Could you check a few things on this drawing? It's one solid part, dimensions in mm from its lowest x, y, z. Round coordinates to 2 decimals unless told otherwise and drop trailing zeros. Write each loop counter-clockwise with the first axis right and the second up, starting at its lowest first coordinate (ties: lowest second). Pieces come first, ordered by that corner, then holes. Notation, with made-up numbers: (5.5, -10.75) -> (56.5, -10.75) arc R29 cw to (56.5, 11.25) -> close; hole circle Ø5 at (70.5, 44). An arc over 180 degrees is marked (long way). Answer in a Markdown table with one row per item.
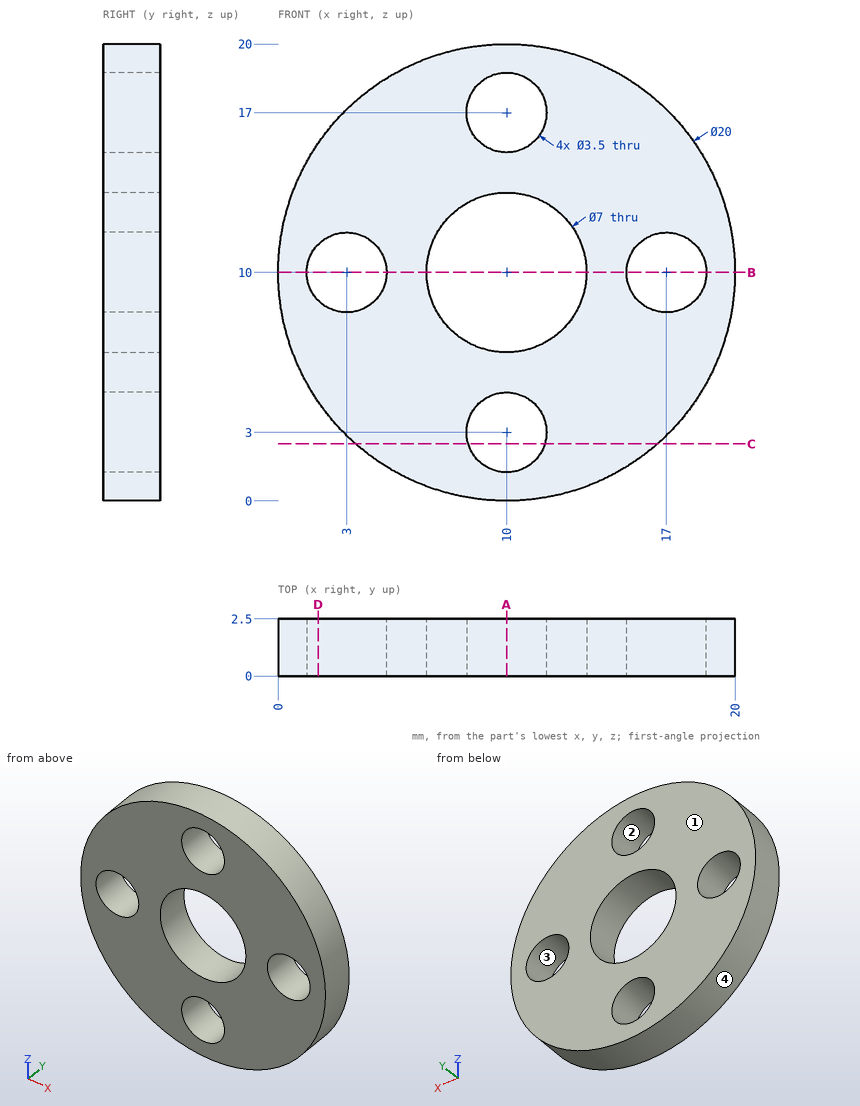
1) Please list where these lines run through material, in increasing order: line 1 (Z direction, x = 10, y = 1); line 2 (X direction, y = 2.3, z = 16).
Findings:
| item | result |
|---|---|
| line 1 | z = 0 to 1.25, 4.75 to 6.5, 13.5 to 15.25, 18.75 to 20 |
| line 2 | x = 2 to 8.56, 11.44 to 18 |
2) Imagine slicing it at A-A, the plane x = 10. Please give me the cut outline in (y, z).
Findings:
| item | result |
|---|---|
| outline | (0, 0) -> (2.5, 0) -> (2.5, 1.25) -> (0, 1.25) -> close; (0, 4.75) -> (2.5, 4.75) -> (2.5, 6.5) -> (0, 6.5) -> close; (0, 13.5) -> (2.5, 13.5) -> (2.5, 15.25) -> (0, 15.25) -> close; (0, 18.75) -> (2.5, 18.75) -> (2.5, 20) -> (0, 20) -> close |
3) For pin 1 (1 mm diameter, centred on x = 15.5, y = 2, fed in from +Z), with a flat end and sliding along its axis, tell me the tip position at first contact or that it passes through.
Findings:
| item | result |
|---|---|
| pin 1 | stops at z = 18.66 |
4) Thinking about a two-plate mould opening in Z: for the marked faces 1, 2, 3 and 4, which applies, +Z half, -Z half, draft (parallel to the pull), parting line (faces both ways), or undercut?
Findings:
| item | result |
|---|---|
| face 1 | draft |
| face 2 | undercut |
| face 3 | undercut |
| face 4 | parting line |
5) Imagine slicing it at B-B, the plane z = 10. Please give me the cut outline in (x, y), plus the area to 3 significant figures.
Findings:
| item | result |
|---|---|
| outline | (0, 0) -> (1.25, 0) -> (1.25, 2.5) -> (0, 2.5) -> close; (4.75, 0) -> (6.5, 0) -> (6.5, 2.5) -> (4.75, 2.5) -> close; (13.5, 0) -> (15.25, 0) -> (15.25, 2.5) -> (13.5, 2.5) -> close; (18.75, 0) -> (20, 0) -> (20, 2.5) -> (18.75, 2.5) -> close |
| area | 15.0 mm^2 |
6) Imagine slicing it at C-C, the plane z = 2.5. Please give me the cut outline in (x, y), plus the area to 3 significant figures.
Findings:
| item | result |
|---|---|
| outline | (3.39, 0) -> (8.32, 0) -> (8.32, 2.5) -> (3.39, 2.5) -> close; (11.68, 0) -> (16.61, 0) -> (16.61, 2.5) -> (11.68, 2.5) -> close |
| area | 24.7 mm^2 |
7) Imagine slicing it at D-D, the plane x = 1.75. Please give me the cut outline in (y, z).
Findings:
| item | result |
|---|---|
| outline | (0, 4.35) -> (2.5, 4.35) -> (2.5, 8.78) -> (0, 8.78) -> close; (0, 11.22) -> (2.5, 11.22) -> (2.5, 15.65) -> (0, 15.65) -> close |
